The model under review builds one solid part; all positions refer to its coordinate system, in mm. A direction names the side the tool comes from. Coordinates: 2 decimals unless noted, no trailing zeros. Loops run counter-clockwise (first coordinate to the right, second up) from the corner with the lowest first, then second, coordinate; pieces in that order, holes last. Notation, with made-up numbers: M 62.25,27.25 L 90.25,27.25 A36 ccw 90.25,63.25 Z; hole C -14,18 d11. An arc over 180 degrees is marked long. Return JSON: item names as keys, results as strings.
Autodesk Inventor part; units mm, degrees
ref_plane "YZ Plane" through (0, 0, 0) normal (1, 0, 0) x (0, 1, 0)
ref_plane "XZ Plane" through (0, 0, 0) normal (0, 1, 0) x (-1, 0, 0)
ref_plane "XY Plane" through (0, 0, 0) normal (0, 0, 1) x (1, 0, 0)
sketch "草圖1" plane through (0, 0, 0) normal (0, 1, 0) x (-1, 0, 0)
  line L0 (0, 0) -> (5, 0)
  line L1 (5, 0) -> (5, -250)
  line L2 (5, -250) -> (0, -250)
  line L3 (0, -250) -> (0, 0)
  dimension "d0" = 5
  dimension "d1" = 250
extrude "擠出1" add sketch "草圖1" along normal blind 15
sketch "草圖3" plane through (0, 15, 0) normal (0, 1, 0) x (1, 0, 0)
  line L0 (0, 250) -> (-5, 250)
  line L1 (0, 0) -> (-5, 0)
  line L2 (-5, 0) -> (-5, 250)
  line L3 (-5, 250) -> (0, 250)
  line L4 (0, 250) -> (0, 0)
extrude "擠出3" add sketch "草圖3" along normal blind 10
sketch "草圖4" plane through (-5, 0, 0) normal (0, 0, 1) x (1, 0, 0)
  line L0 (5, 0) -> (5, 25)
  line L1 (0, 25) -> (5, 25)
  line L2 (5, 25) -> (0, 25)
  line L3 (5, 25) -> (25, 35)
  line L4 (5, 15) -> (25, 5)
  line L5 (25, 5) -> (25, 35)
  line L6 (0, 0) -> (5, 0)
  line L7 (0, 0) -> (0, 25)
  line L8 (-5, 0) -> (30, 0)
  dimension "d8" = 10
  dimension "d9" = 30
  dimension "d19" = 20
extrude "擠出4" add sketch "草圖4" against normal up to surface (250 mm away) contours L0 L3 L5 L4
shell "薄殼2" thickness 1 removed faces 2 at (20, 15, -83.3333) at (-1.6667, 0, -83.3333)
equation "\"d0\" = bottom_w"
equation "\"d1\" = bottom_l"
equation "\"d2\" = bottom_h"
equation "\"d6\" = nuzzle_lh"
equation "\"d8\" = nuzzle_lh"
equation "\"d9\" = 3 * nuzzle_lh"
equation "\"d15\" = nuzzle_lh"
equation "\"bottom_w\" = 5"
equation "\"bottom_l\" = 250"
equation "\"bottom_h\" = 15"
equation "\"nuzzle_lh\" = 10"
properties part number "nuzzle_v1_0310"
1. Add section A-A on z = -97. Give the boundary of the cut face in (x, y).
Check values:
{"outline": "M -5,0 L -4,0 L -4,24 L 0.24,24 L 20,33.88 L 20,35 L 0,25 L -5,25 Z; M -1,0 L 0,0 L 0,15 L 20,5 L 20,6.12 L -1,16.62 Z"}
2. The part is to be moulded in two halves that separate along Z. For faces 1 (the face through (-2, 24, -127)), 2 (the face through (7, 18, 0)), 3 (the face through (0, 7, -127)), say which applies: released by +Z, released by -Z, zero draft, split by the parting line, or undercut.
Check values:
{"face 1": "undercut", "face 2": "released by +Z", "face 3": "zero draft"}
3. Insertion check: pin 1 Ø3 at (y, z) = (22, -159.5) entering from +X; pin 2 Ø4 at (x, z) = (2.5, -186.5) entering from +Y; pin 3 Ø6 at (x, z) = (10, -126) entering from +Y. Each pin has a flat end and moves straight along its axis. Give the tip position at first contact, or say it passes through.
Check values:
{"pin 1": "x = -4", "pin 2": "y = 27.25", "pin 3": "y = 31.5"}
4. To check wall thickness, follow line 1 (Z direction, x = 0, y = 22.5); line 2 (X direction, y = 13, z = -18.5); line 3 (X direction, y = 4, z = -187.5). State the ranges of each line that lie inside material, in increasing order.
Check values:
{"line 1": "-250 to -249, -1 to 0", "line 2": "-5 to -4, -1 to 0, 4 to 6.24", "line 3": "-5 to -4, -1 to 0"}
5. Add section B-B on x = 10.5. Give the boundary of the cut face in (y, z), plus the area to 3 significant figures.
Check values:
{"outline": "M 9.75,-250 L 30.25,-250 L 30.25,0 L 9.75,0 Z; hole M 10.87,-249 L 29.13,-249 L 29.13,-1 L 10.87,-1 Z", "area": "596 mm²"}
6. Machinability: for faces 4 (the face through (-3, 25, -127)), 5 (the face through (-0.8, 0, -123.2)), 6 (the face through (-1, 8, -127)), 7 (the face through (10, 10, -123)), 8 (the face through (9.353, 11.442, -123.264)), which of the approach directions +Z, -Z, +X, -X, +Y, -Y give a long, thin tool a straight path to every point of the face, cutting with its end or side? Answer none if there is none.
Check values:
{"face 4": "+Z, -Z, -X, +Y", "face 5": "+Z, -Z, +X, -X, -Y", "face 6": "-Y", "face 7": "+Z, -Z, -Y", "face 8": "+X"}
7. Add section C-C on y = 30. Give the boundary of the cut face in (x, z), plus the area to 3 significant figures.
Check values:
{"outline": "M 10,-250 L 20,-250 L 20,-249 L 12.24,-249 L 12.24,-1 L 20,-1 L 20,0 L 10,0 Z", "area": "575 mm²"}
